```python
from build123d import *

# Parameters (mm, degrees)
F0_R     = 2
F1_DEPTH = 5
F2_R     = 5
F3_DEPTH = 10
F4_SIZE  = 1


with BuildPart() as f1:
    # F0 (on Top) → F1 (new body)
    with BuildSketch(Plane.XY):
        Polygon((16.2357693204, 0.0607577779), (11.4374603474, 11.523384821), (-0.0607577779, 16.2357693204), (-11.523384821, 11.4374603474), (-16.2357693204, -0.0607577779), (-11.4374603474, -11.523384821), (0.0607577779, -16.2357693204), (11.523384821, -11.4374603474), align=None)
        Circle(F0_R, mode=Mode.SUBTRACT)
    extrude(amount=F1_DEPTH)

    # F2 (on face) → F3 (join)
    with BuildSketch(Plane.XY.offset(5)):
        Circle(F2_R)
        with BuildLine():
            Line((0.9682458366, 1.75), (1.75, 1.75))
            Line((1.75, 1.75), (1.75, 0.9682458366))
            ThreePointArc((1.75, 0.9682458366), (1.9364916731, 0.5), (2, 0))
            ThreePointArc((2, 0), (1.9364916731, -0.5), (1.75, -0.9682458366))
            Line((1.75, -0.9682458366), (1.75, -1.75))
            Line((1.75, -1.75), (0.9682458366, -1.75))
            ThreePointArc((0.9682458366, -1.75), (0, -2), (-0.9682458366, -1.75))
            Line((-0.9682458366, -1.75), (-1.75, -1.75))
            Line((-1.75, -1.75), (-1.75, -0.9682458366))
            ThreePointArc((-1.75, -0.9682458366), (-2, 0), (-1.75, 0.9682458366))
            Line((-1.75, 0.9682458366), (-1.75, 1.75))
            Line((-1.75, 1.75), (-0.9682458366, 1.75))
            ThreePointArc((-0.9682458366, 1.75), (0, 2), (0.9682458366, 1.75))
        make_face(mode=Mode.SUBTRACT)
        with BuildLine():
            Line((-0.9682458366, 1.75), (0.9682458366, 1.75))
            ThreePointArc((0.9682458366, 1.75), (0, 2), (-0.9682458366, 1.75))
        make_face()
        with BuildLine():
            ThreePointArc((2, 0), (1.9364916731, 0.5), (1.75, 0.9682458366))
            Line((1.75, 0.9682458366), (1.75, -0.9682458366))
            ThreePointArc((1.75, -0.9682458366), (1.9364916731, -0.5), (2, 0))
        make_face()
        with BuildLine():
            ThreePointArc((-0.9682458366, -1.75), (0, -2), (0.9682458366, -1.75))
            Line((0.9682458366, -1.75), (-0.9682458366, -1.75))
        make_face()
        with BuildLine():
            Line((-1.75, -0.9682458366), (-1.75, 0.9682458366))
            ThreePointArc((-1.75, 0.9682458366), (-2, 0), (-1.75, -0.9682458366))
        make_face()
    extrude(amount=F3_DEPTH)

    # F4
    f4_edges = [f1.edges().sort_by_distance(p)[0] for p in [
        (-5, 0, 15),
        (0, 1.75, 15),
        (1.75, 0, 15),
        (0, -1.75, 15),
        (-1.75, 0, 15),
        (-5, 0, 5),
        (13.879577, -5.688351, 5),
        (13.836615, 5.792071, 5),
        (5.792071, -13.836615, 5),
        (-5.688351, -13.879577, 5),
        (5.688351, 13.879577, 5),
        (-13.836615, -5.792071, 5),
        (-5.792071, 13.836615, 5),
        (-13.879577, 5.688351, 5),
        (13.879577, -5.688351, 0),
        (13.836615, 5.792071, 0),
        (5.688351, 13.879577, 0),
        (-5.792071, 13.836615, 0),
        (-13.879577, 5.688351, 0),
        (-13.836615, -5.792071, 0),
        (-5.688351, -13.879577, 0),
        (5.792071, -13.836615, 0),
        (-2, 0, 0),
    ]]
    chamfer(f4_edges, length=F4_SIZE)


solid = f1.part
```
For this review, take the finished solid that the model builds, in its own axes (mm). A direction names the side the tool comes from. Round coordinates to 2 decimals unless told otherwise and drop trailing zeros. Write each loop counter-clockwise with the first axis right and the second up, starting at its lowest first coordinate (ties: lowest second). Pieces come first, ordered by that corner, then holes. Notation, with made-up numbers: (66, -1.5) - (80, -1.5) arc R20 cw to (80, 3.5) - close; hole circle Ø9 at (-38.5, 51). An arc over 180 degrees is marked (long way). Put each result on its own line as item: value.
Q1. Machinability: for faces 4 (the face through (-13.377, 5.577, 0.493)), 5 (the face through (0, 1.75, 9)), which of the approach directions +Z, -Z, +X, -X, +Y, -Y give a long, thin tool a straight path to every point of the face, cutting with its end or side? Answer none if there is none.
Solved:
face 4: -Z, -X, +Y
face 5: +Z
Q2. Wall thickness on probe 1 along Z at (x, y) = (-9, -0.5); probe 2 along Y at (x, z) = (0, 3.1); probe 3 along X at (y, z) = (-4, 8.5): over which ranges is each line inside the solid? List them lowest first.
Solved:
probe 1: z = 0 to 5
probe 2: y = -16.21 to -2, 2 to 16.21
probe 3: x = -3 to 3
Q3. We need section C-C (x = 10). Give the boundary of the cut face in (y, z), and give its area (3 significant figures).
Solved:
outline: (-12.08, 1) - (-10.99, 0) - (11.03, 0) - (12.11, 1) - (12.11, 4) - (11.03, 5) - (-10.99, 5) - (-12.08, 4) - close
area: 119 mm2
Q4. We need section B-B (y = 7.5). Give the boundary of the cut face in (x, z), and give its area (3 significant figures).
Solved:
outline: (-13.14, 1) - (-12.06, 0) - (12.04, 0) - (13.12, 1) - (13.12, 4) - (12.04, 5) - (-12.06, 5) - (-13.14, 4) - close
area: 129 mm2
Q5. Insertion check: pin 1 Ø8 at (y, z) = (0.5, 13) entering from -X; pin 2 Ø0.9 at (x, y) = (1.5, 1.5) entering from +Z; pin 3 Ø1 at (x, z) = (-4, 11) entering from -Y. Each pin has a flat end and moves straight along its axis. Give the tip position at first contact, or say it passes through.
Solved:
pin 1: stops at x = -5
pin 2: stops at z = 14.2
pin 3: stops at y = -3.57
Q6. We need section A-A (z = 7.25). Give the boundary of the cut face in (x, y).
Solved:
outline: circle Ø10 at (0, 0); hole (-1.75, -1.75) - (1.75, -1.75) - (1.75, 1.75) - (-1.75, 1.75) - close
Q7. Mouldability with a two-part tool opening along Y and no side actions: class faces 1 (the face through (-1.08, -4.88, 9.94)), 2 (the face through (0, -1.75, 9)), 3 (the face through (0, -7, 5)) as released by +Y, released by -Y, zero draft, split by the parting line, or undercut.
Solved:
face 1: split by the parting line
face 2: undercut
face 3: zero draft
